Geometry: final body of the model. Coordinates: model frame, mm. Coordinates: 2 decimals unless noted, no trailing zeros. Put each result on its own line as item: value.
```python
from build123d import *

# Parameters (mm, degrees)
CYLINDER012029001078_R     = 1.75
CYLINDER012029001078_DEPTH = 4
CYLINDER012029001079_R     = 1.75
CYLINDER012029001079_DEPTH = 4
CYLINDER012029001080_R     = 1.75
CYLINDER012029001080_DEPTH = 4
CYLINDER012029001077_R     = 1.75
CYLINDER012029001077_DEPTH = 4
CYLINDER021_R              = 1.6
CYLINDER021_DEPTH          = 10
CYLINDER020_R              = 1.6
CYLINDER020_DEPTH          = 10
CYLINDER019_R              = 1.6
CYLINDER019_DEPTH          = 10
CYLINDER018_R              = 1.6
CYLINDER018_DEPTH          = 10
CYLINDER017_R              = 1.6
CYLINDER017_DEPTH          = 10
CYLINDER016_R              = 1.6
CYLINDER016_DEPTH          = 10
CYLINDER015_R              = 1.6
CYLINDER015_DEPTH          = 10
CYLINDER014_R              = 1.6
CYLINDER014_DEPTH          = 10
CYLINDER013_R              = 5.6
CYLINDER013_DEPTH          = 10
CYLINDER012029001069_R     = 1.6
CYLINDER012029001069_DEPTH = 10
CYLINDER012029001070_R     = 1.6
CYLINDER012029001070_DEPTH = 10
CYLINDER012029001071_R     = 1.6
CYLINDER012029001071_DEPTH = 10
CYLINDER012029001072_R     = 1.6
CYLINDER012029001072_DEPTH = 10
CYLINDER012029001073_R     = 1.6
CYLINDER012029001073_DEPTH = 10
CYLINDER012029001074_R     = 5.6
CYLINDER012029001074_DEPTH = 10
CYLINDER012029001068_R     = 1.6
CYLINDER012029001068_DEPTH = 10
CYLINDER012029001067_R     = 1.6
CYLINDER012029001067_DEPTH = 10
CYLINDER012029001066_R     = 1.6
CYLINDER012029001066_DEPTH = 10
CYLINDER012029001062_R     = 7.6
CYLINDER012029001062_DEPTH = 10
CYLINDER012029001065_R     = 7.6
CYLINDER012029001065_DEPTH = 10
CYLINDER012029001063_R     = 7.6
CYLINDER012029001063_DEPTH = 10
CYLINDER012029001064_R     = 7.6
CYLINDER012029001064_DEPTH = 10
BOX015001052_W             = 368
BOX015001052_H             = 241
BOX015001052_DEPTH         = 4


with BuildPart() as cylinder012029001081:
    # Cylinder012029001078 → Cylinder012029001078 (new body)
    with BuildSketch(Plane(origin=(75.63, 233.64, 0), x_dir=(1, 0, 0), z_dir=(0, 0, 1))):
        Circle(CYLINDER012029001078_R)
    extrude(amount=CYLINDER012029001078_DEPTH)


with BuildPart() as cylinder012029001082:
    # Cylinder012029001079 → Cylinder012029001079 (new body)
    with BuildSketch(Plane(origin=(284.37, 233.64, 0), x_dir=(1, 0, 0), z_dir=(0, 0, 1))):
        Circle(CYLINDER012029001079_R)
    extrude(amount=CYLINDER012029001079_DEPTH)


with BuildPart() as cylinder012029001083:
    # Cylinder012029001080 → Cylinder012029001080 (new body)
    with BuildSketch(Plane(origin=(284.37, 26.63, 0), x_dir=(1, 0, 0), z_dir=(0, 0, 1))):
        Circle(CYLINDER012029001080_R)
    extrude(amount=CYLINDER012029001080_DEPTH)


with BuildPart() as fusion001019007006:
    # Cylinder012029001077 → Cylinder012029001077 (new body)
    with BuildSketch(Plane(origin=(75.63, 26.63, 0), x_dir=(1, 0, 0), z_dir=(0, 0, 1))):
        Circle(CYLINDER012029001077_R)
    extrude(amount=CYLINDER012029001077_DEPTH)

    # Fusion001019007006: union Cylinder012029001081, Cylinder012029001082, Cylinder012029001083
    add(cylinder012029001081.part)
    add(cylinder012029001082.part)
    add(cylinder012029001083.part)


with BuildPart() as cylinder022:
    # Cylinder021 → Cylinder021 (new body)
    with BuildSketch(Plane(origin=(338, 25, -1), x_dir=(1, 0, 0), z_dir=(0, 0, 1))):
        Circle(CYLINDER021_R)
    extrude(amount=CYLINDER021_DEPTH)


with BuildPart() as cylinder021:
    # Cylinder020 → Cylinder020 (new body)
    with BuildSketch(Plane(origin=(338, 49, -1), x_dir=(1, 0, 0), z_dir=(0, 0, 1))):
        Circle(CYLINDER020_R)
    extrude(amount=CYLINDER020_DEPTH)


with BuildPart() as cylinder020:
    # Cylinder019 → Cylinder019 (new body)
    with BuildSketch(Plane(origin=(338, 192, -1), x_dir=(1, 0, 0), z_dir=(0, 0, 1))):
        Circle(CYLINDER019_R)
    extrude(amount=CYLINDER019_DEPTH)


with BuildPart() as cylinder019:
    # Cylinder018 → Cylinder018 (new body)
    with BuildSketch(Plane(origin=(338, 216, -1), x_dir=(1, 0, 0), z_dir=(0, 0, 1))):
        Circle(CYLINDER018_R)
    extrude(amount=CYLINDER018_DEPTH)


with BuildPart() as cylinder018:
    # Cylinder017 → Cylinder017 (new body)
    with BuildSketch(Plane(origin=(349, 128.5, -1), x_dir=(1, 0, 0), z_dir=(0, 0, 1))):
        Circle(CYLINDER017_R)
    extrude(amount=CYLINDER017_DEPTH)


with BuildPart() as cylinder012029001078:
    # Cylinder016 → Cylinder016 (new body)
    with BuildSketch(Plane(origin=(349, 112.5, -1), x_dir=(1, 0, 0), z_dir=(0, 0, 1))):
        Circle(CYLINDER016_R)
    extrude(amount=CYLINDER016_DEPTH)


with BuildPart() as cylinder012029001079:
    # Cylinder015 → Cylinder015 (new body)
    with BuildSketch(Plane(origin=(357, 120.5, -1), x_dir=(1, 0, 0), z_dir=(0, 0, 1))):
        Circle(CYLINDER015_R)
    extrude(amount=CYLINDER015_DEPTH)


with BuildPart() as cylinder012029001077:
    # Cylinder014 → Cylinder014 (new body)
    with BuildSketch(Plane(origin=(341, 120.5, -1), x_dir=(1, 0, 0), z_dir=(0, 0, 1))):
        Circle(CYLINDER014_R)
    extrude(amount=CYLINDER014_DEPTH)


with BuildPart() as cylinder012029001076:
    # Cylinder013 → Cylinder013 (new body)
    with BuildSketch(Plane(origin=(349, 120.5, -1), x_dir=(1, 0, 0), z_dir=(0, 0, 1))):
        Circle(CYLINDER013_R)
    extrude(amount=CYLINDER013_DEPTH)


with BuildPart() as cylinder012029001070:
    # Cylinder012029001069 → Cylinder012029001069 (new body)
    with BuildSketch(Plane(origin=(22, 216, -1), x_dir=(1, 0, 0), z_dir=(0, 0, 1))):
        Circle(CYLINDER012029001069_R)
    extrude(amount=CYLINDER012029001069_DEPTH)


with BuildPart() as cylinder012029001071:
    # Cylinder012029001070 → Cylinder012029001070 (new body)
    with BuildSketch(Plane(origin=(11, 112.5, -1), x_dir=(1, 0, 0), z_dir=(0, 0, 1))):
        Circle(CYLINDER012029001070_R)
    extrude(amount=CYLINDER012029001070_DEPTH)


with BuildPart() as cylinder012029001072:
    # Cylinder012029001071 → Cylinder012029001071 (new body)
    with BuildSketch(Plane(origin=(19, 120.5, -1), x_dir=(1, 0, 0), z_dir=(0, 0, 1))):
        Circle(CYLINDER012029001071_R)
    extrude(amount=CYLINDER012029001071_DEPTH)


with BuildPart() as cylinder012029001073:
    # Cylinder012029001072 → Cylinder012029001072 (new body)
    with BuildSketch(Plane(origin=(11, 128.5, -1), x_dir=(1, 0, 0), z_dir=(0, 0, 1))):
        Circle(CYLINDER012029001072_R)
    extrude(amount=CYLINDER012029001072_DEPTH)


with BuildPart() as cylinder012029001074:
    # Cylinder012029001073 → Cylinder012029001073 (new body)
    with BuildSketch(Plane(origin=(3, 120.5, -1), x_dir=(1, 0, 0), z_dir=(0, 0, 1))):
        Circle(CYLINDER012029001073_R)
    extrude(amount=CYLINDER012029001073_DEPTH)


with BuildPart() as cylinder012029001075:
    # Cylinder012029001074 → Cylinder012029001074 (new body)
    with BuildSketch(Plane(origin=(11, 120.5, -1), x_dir=(1, 0, 0), z_dir=(0, 0, 1))):
        Circle(CYLINDER012029001074_R)
    extrude(amount=CYLINDER012029001074_DEPTH)


with BuildPart() as cylinder012029001069:
    # Cylinder012029001068 → Cylinder012029001068 (new body)
    with BuildSketch(Plane(origin=(22, 192, -1), x_dir=(1, 0, 0), z_dir=(0, 0, 1))):
        Circle(CYLINDER012029001068_R)
    extrude(amount=CYLINDER012029001068_DEPTH)


with BuildPart() as cylinder012029001068:
    # Cylinder012029001067 → Cylinder012029001067 (new body)
    with BuildSketch(Plane(origin=(22, 49, -1), x_dir=(1, 0, 0), z_dir=(0, 0, 1))):
        Circle(CYLINDER012029001067_R)
    extrude(amount=CYLINDER012029001067_DEPTH)


with BuildPart() as cylinder012029001067:
    # Cylinder012029001066 → Cylinder012029001066 (new body)
    with BuildSketch(Plane(origin=(22, 25, -1), x_dir=(1, 0, 0), z_dir=(0, 0, 1))):
        Circle(CYLINDER012029001066_R)
    extrude(amount=CYLINDER012029001066_DEPTH)


with BuildPart() as cylinder012029001066:
    # Cylinder012029001062 → Cylinder012029001062 (new body)
    with BuildSketch(Plane(origin=(338, 204, -1), x_dir=(1, 0, 0), z_dir=(0, 0, 1))):
        Circle(CYLINDER012029001062_R)
    extrude(amount=CYLINDER012029001062_DEPTH)


with BuildPart() as cylinder012029001065:
    # Cylinder012029001065 → Cylinder012029001065 (new body)
    with BuildSketch(Plane(origin=(338, 37, -1), x_dir=(1, 0, 0), z_dir=(0, 0, 1))):
        Circle(CYLINDER012029001065_R)
    extrude(amount=CYLINDER012029001065_DEPTH)


with BuildPart() as cylinder012029001063:
    # Cylinder012029001063 → Cylinder012029001063 (new body)
    with BuildSketch(Plane(origin=(22, 204, -1), x_dir=(1, 0, 0), z_dir=(0, 0, 1))):
        Circle(CYLINDER012029001063_R)
    extrude(amount=CYLINDER012029001063_DEPTH)


with BuildPart() as cylinder012029001064:
    # Cylinder012029001064 → Cylinder012029001064 (new body)
    with BuildSketch(Plane(origin=(22, 37, -1), x_dir=(1, 0, 0), z_dir=(0, 0, 1))):
        Circle(CYLINDER012029001064_R)
    extrude(amount=CYLINDER012029001064_DEPTH)


with BuildPart() as cut003059:
    # Box015001052 → Box015001052 (new body)
    with BuildSketch(Plane(origin=(-4, 0, 0), x_dir=(1, 0, 0), z_dir=(0, 0, 1))):
        with Locations((184, 120.5)):
            Rectangle(BOX015001052_W, BOX015001052_H)
    extrude(amount=BOX015001052_DEPTH)

    # Cut003058: cut Cylinder012029001064
    add(cylinder012029001064.part, mode=Mode.SUBTRACT)

    # Cut003055: cut Cylinder012029001063
    add(cylinder012029001063.part, mode=Mode.SUBTRACT)

    # Cut003057: cut Cylinder012029001065
    add(cylinder012029001065.part, mode=Mode.SUBTRACT)

    # Cut003056: cut Cylinder012029001066
    add(cylinder012029001066.part, mode=Mode.SUBTRACT)

    # Cut004: cut Cylinder012029001067
    add(cylinder012029001067.part, mode=Mode.SUBTRACT)

    # Cut005: cut Cylinder012029001068
    add(cylinder012029001068.part, mode=Mode.SUBTRACT)

    # Cut006: cut Cylinder012029001069
    add(cylinder012029001069.part, mode=Mode.SUBTRACT)

    # Cut007: cut Cylinder012029001075
    add(cylinder012029001075.part, mode=Mode.SUBTRACT)

    # Cut008: cut Cylinder012029001074
    add(cylinder012029001074.part, mode=Mode.SUBTRACT)

    # Cut009: cut Cylinder012029001073
    add(cylinder012029001073.part, mode=Mode.SUBTRACT)

    # Cut010: cut Cylinder012029001072
    add(cylinder012029001072.part, mode=Mode.SUBTRACT)

    # Cut011: cut Cylinder012029001071
    add(cylinder012029001071.part, mode=Mode.SUBTRACT)

    # Cut012: cut Cylinder012029001070
    add(cylinder012029001070.part, mode=Mode.SUBTRACT)

    # Cut013: cut Cylinder012029001076
    add(cylinder012029001076.part, mode=Mode.SUBTRACT)

    # Cut014: cut Cylinder012029001077
    add(cylinder012029001077.part, mode=Mode.SUBTRACT)

    # Cut015: cut Cylinder012029001079
    add(cylinder012029001079.part, mode=Mode.SUBTRACT)

    # Cut016: cut Cylinder012029001078
    add(cylinder012029001078.part, mode=Mode.SUBTRACT)

    # Cut017: cut Cylinder018
    add(cylinder018.part, mode=Mode.SUBTRACT)

    # Cut018: cut Cylinder019
    add(cylinder019.part, mode=Mode.SUBTRACT)

    # Cut019: cut Cylinder020
    add(cylinder020.part, mode=Mode.SUBTRACT)

    # Cut020: cut Cylinder021
    add(cylinder021.part, mode=Mode.SUBTRACT)

    # Cut021: cut Cylinder022
    add(cylinder022.part, mode=Mode.SUBTRACT)

    # Cut003059: cut Fusion001019007006
    add(fusion001019007006.part, mode=Mode.SUBTRACT)


solid = cut003059.part
```
1. Ray query, probe 1 along X at (y, z) = (203, 1.75); probe 2 along Y at (x, z) = (11, 3); probe 3 along X at (y, z) = (49, 1.95). Return the intervals inside material, ascending. Write a range as from..to.
Answer below:
probe 1: x = -4..14.47, 29.53..330.47, 345.53..364
probe 2: y = 0..110.9, 114.1..114.9, 126.1..126.9, 130.1..241
probe 3: x = -4..20.4, 23.6..336.4, 339.6..364
2. Mould query, pull axis X, two halves, no side actions, for faces 1 (the cylindrical face through (20.35, 196.58, 1.97)), 2 (the flat face through (177, 122, 0)). Classes: +X half, -X half, draft (parallel to the pull), parting line (faces both ways), or undercut.
Answer below:
face 1: undercut
face 2: draft
3. Pin query (flat end, axial travel): pin 1 Ø1.9 at (x, y) = (11, 128.5) entering from -Z. Return the tip coordinate at first contact, or that it passes through.
Answer below:
pin 1: passes through
